Read the model definition and answer for the solid it produces. Units are mm, in the model's axes. Round coordinates to 2 decimals unless told otherwise and drop trailing zeros. Loops run counter-clockwise (first coordinate to the right, second up) from the corner with the lowest first, then second, coordinate; pieces in that order, holes last. Notation, with made-up numbers: (45, -31.5) -> (91, -31.5) arc R15 cw to (91, -19.5) -> close; hole circle Ø3 at (69.25, 80). An arc over 180 degrees is marked (long way). Put each result on its own line as item: value.
from build123d import *

# Parameters (mm, degrees)
F2_DEPTH = 25.4
F3_DEPTH = 9.398


with BuildPart() as f1:
    # F0 (on Front) → F1 (revolve)
    with BuildSketch(Plane.XZ):
        Polygon((11.2185701728, 72.9290992022), (159.1500639915, 72.9290992022), (10, 131.0742050409), (0, 131.0742050409), (0, 128.5420060158), (10.000754334, 128.5420060158), (135.111038288, 79.7686397339), (11.2185701728, 79.6332210302), align=None)
    revolve(axis=Axis((0, 0, 129.8081055284), (0, 0, 1)))

    # F2 (cut): a face of the model
    f2_faces = [f1.faces().sort_by_distance(p)[0] for p in [
        (0, 0, 131.0742050409),
    ]]
    extrude(f2_faces, amount=-F2_DEPTH, mode=Mode.SUBTRACT)

    # F3 (cut): a face of the model
    f3_faces = [f1.faces().sort_by_distance(p)[0] for p in [
        (-15.7200137518, 0, 72.9290992022),
    ]]
    extrude(f3_faces, amount=-F3_DEPTH, mode=Mode.SUBTRACT)


solid = f1.part
Item 1: The part is cut by section C-C (z = 108.5). Determine the outline of the cut face in (x, y), then the cut area to 3 significant figures.
Derived:
outline: circle Ø135.81 at (0, 0); hole circle Ø122.82 at (0, 0)
area: 2,640 mm^2
Item 2: For a pull along X with two mould halves and no side action, classify faces 1 (the flat face through (-119.4, -49.4, 82.327)), 2 (the cylindrical face through (-2.17, -9.76, 129.83)), 3 (the conical face through (15.329, 4.827, 128.707)) as pulls with the +X half, pulls with the -X half, needs draft (parallel to the pull), parting line crosses it, or undercut.
Derived:
face 1: needs draft
face 2: undercut
face 3: parting line crosses it
Item 3: Flat-ended cylindrical pins translate along their axes: pin 1 Ø1.5 at (x, y) = (-68.5, 105.5) entering from +Z; pin 2 Ø10 at (y, z) = (-73, 115.5) entering from -X. Find the tip coordinate at first contact, or state that the pin passes through.
Derived:
pin 1: stops at z = 86.23
pin 2: passes through
Item 4: Find the intervals of material crossed by line 1 along Z through (x, y) = (-14.5, 65.5); line 2 along Z through (x, y) = (-50, -3), in increasing order.
Derived:
line 1: z = 106.29 to 108.82
line 2: z = 112.91 to 115.45
